```python
from build123d import *

# Parameters (mm, degrees)
SKETCH1_W           = 200
SKETCH1_H           = 90
BOSS_EXTRUDE1_DEPTH = 20
FILLET1_R           = 5
SKETCH2_W           = 25
SKETCH2_H           = 30
BOSS_EXTRUDE2_DEPTH = 14.8
FILLET2_R           = 5
CUT_EXTRUDE1_DEPTH  = 10
CUT_EXTRUDE2_REACH  = 150.214
SKETCH4_R           = 2.5


with BuildPart() as part:
    # Sketch1 → Boss-Extrude1 (new body)
    with BuildSketch(Plane(origin=(0, 0, 0), x_dir=(1, 0, 0), z_dir=(0, 1, 0))):
        with Locations((100, 45)):
            Rectangle(SKETCH1_W, SKETCH1_H)
    extrude(amount=BOSS_EXTRUDE1_DEPTH)

    # Fillet1
    fillet1_edges = [part.edges().sort_by_distance(p)[0] for p in [
        (0, 10, -90),
        (200, 10, -90),
        (200, 10, 0),
        (0, 10, 0),
    ]]
    fillet(fillet1_edges, radius=FILLET1_R)

    # Sketch2 → Boss-Extrude2 (add)
    with BuildSketch(Plane(origin=(0, 20, 0), x_dir=(1, 0, 0), z_dir=(0, 1, 0))):
        with Locations((100, 45)):
            Rectangle(SKETCH2_W, SKETCH2_H)
    extrude(amount=BOSS_EXTRUDE2_DEPTH)

    # Fillet2
    fillet2_edges = [part.edges().sort_by_distance(p)[0] for p in [
        (100, 34.8, -30),
        (100, 34.8, -60),
    ]]
    fillet(fillet2_edges, radius=FILLET2_R)

    # Sketch3 → Cut-Extrude1 (cut)
    with BuildSketch(Plane.ZY.offset(-87.5)):
        Polygon((-49.561067127, 28), (-47.280533563, 24.05), (-42.719466437, 24.05), (-40.438932873, 28), (-42.719466437, 31.95), (-47.280533563, 31.95), align=None)
    extrude(amount=-CUT_EXTRUDE1_DEPTH, mode=Mode.SUBTRACT)

    # Sketch4 → Cut-Extrude2 (cut, up to next)
    with BuildSketch(Plane.ZY.offset(-87.5), mode=Mode.PRIVATE) as cut_extrude2_sk1:
        with Locations((-45, 28)):
            Circle(SKETCH4_R)
    cut_extrude2_tool1 = extrude(cut_extrude2_sk1.sketch, amount=-CUT_EXTRUDE2_REACH, mode=Mode.PRIVATE) & part.part
    add(cut_extrude2_tool1.solids().sort_by_distance((87.5, 28, -45))[0], mode=Mode.SUBTRACT)


solid = part.part
```
Input: part model. Units: mm. Frame: model coordinates. A direction names the side the tool comes from. Coordinates: 2 decimals unless noted, no trailing zeros. Loops run counter-clockwise (first coordinate to the right, second up) from the corner with the lowest first, then second, coordinate; pieces in that order, holes last.
Q1. Section B-B, the plane z = -32. Return the cut outline in (x, y).
Results are:
outline: (0, 0) - (200, 0) - (200, 20) - (112.5, 20) - (112.5, 33.8) - (87.5, 33.8) - (87.5, 20) - (0, 20) - close
Q2. Set-up query: faces 4 (the flat face through (112.5, 24, -45)), 5 (the flat face through (92, 24.05, -45)), 6 (the flat face through (100, 25, -30)), 7 (the flat face through (87.5, 26, -41)). Return all of +Z, -Z, +X, -X, +Y, -Y with unobstructed straight access to the full face (end or side cutting, diameter ignored); none if empty.
Results are:
face 4: +Z, -Z, +X, +Y
face 5: -X
face 6: +Z, +X, -X, +Y
face 7: +Z, -Z, -X, +Y
Q3. Section A-A, the plane z = -45. Return the cut outline in (x, y).
Results are:
outline: (0, 0) - (200, 0) - (200, 20) - (112.5, 20) - (112.5, 25.5) - (97.5, 25.5) - (97.5, 24.05) - (87.5, 24.05) - (87.5, 20) - (0, 20) - close; (87.5, 31.95) - (97.5, 31.95) - (97.5, 30.5) - (112.5, 30.5) - (112.5, 34.8) - (87.5, 34.8) - close
Q4. Section D-D, the plane z = -11.5. Return the cut outline in (x, y).
Results are:
outline: (0, 0) - (200, 0) - (200, 20) - (0, 20) - close
Q5. Contact query for flat-ended pins moving along their axis: pin 1 (3 mm diameter, centred on x = 87, y = 26.5, fed in from +Z); pin 2 (4.5 mm diameter, centred on y = 28, z = -48, fed in from +X); pin 3 (2.5 mm diameter, centred on y = 29, z = -43.5, fed in from -X). Output: stop coordinate, or through.
Results are:
pin 1: stops at z = -30
pin 2: stops at x = 112.5
pin 3: stops at x = 97.5
Q6. Mould query, pull axis Y, two halves, no side actions, for faces 1 (the flat face through (92.43, 25.997, -41.595)), 2 (the cylindrical face through (1, 10, -88)), 3 (the cylindrical face through (100.18, 33.3, -31.43)). Classes: +Y half, -Y half, draft (parallel to the pull), parting line (faces both ways), or undercut.
Results are:
face 1: undercut
face 2: draft
face 3: +Y half
Q7. Section C-C, the plane x = 71. Return the cut outline in (y, z), and give its area (3 significant figures).
Results are:
outline: (0, -90) - (20, -90) - (20, 0) - (0, 0) - close
area: 1,800 mm2
Q8. Line query: line 1 along Y through (x, z) = (105.75, -45); line 2 along X through (y, z) = (28, -42); line 3 along Y through (x, z) = (57.5, -11.5). Output: solid intervals per line, ascending.
Results are:
line 1: y = 0 to 25.5, 30.5 to 34.8
line 2: x = 97.5 to 112.5
line 3: y = 0 to 20
